from build123d import *

# Parameters (mm, degrees)
BOSS_EXTRUDE1_DEPTH = 2


with BuildPart() as part:
    # Sketch2 → Boss-Extrude1 (new body)
    with BuildSketch(Plane(origin=(0, 0, 0), x_dir=(1, 0, 0), z_dir=(0, 1, 0))):
        with BuildLine():
            Line((-3.625231148, -1.690473047), (-2.357376363, -4.409396408))
            ThreePointArc((-2.357376363, -4.409396408), (-1.93416063, -4.797202177), (-1.360681826, -4.772163552))
            Line((-1.360681826, -4.772163552), (-1.13410488, -4.666508987))
            ThreePointArc((-1.13410488, -4.666508987), (-0.96265902, -4.513901105), (-0.903326596, -4.292174896))
            Line((-0.903326596, -4.292174896), (-0.941712266, -2.992741735))
            ThreePointArc((-0.941712266, -2.992741735), (-1.04172473, -2.435992925), (-1.3, -1.932737905))
            ThreePointArc((-1.3, -1.932737905), (0, 0.6), (1.3, -1.932737905))
            ThreePointArc((1.3, -1.932737905), (1.04172473, -2.435992925), (0.941712266, -2.992741735))
            Line((0.941712266, -2.992741735), (0.903326596, -4.292174896))
            ThreePointArc((0.903326596, -4.292174896), (0.96265902, -4.513901105), (1.13410488, -4.666508987))
            Line((1.13410488, -4.666508987), (1.360681826, -4.772163552))
            ThreePointArc((1.360681826, -4.772163552), (1.93416063, -4.797202177), (2.357376363, -4.409396408))
            Line((2.357376363, -4.409396408), (3.625231148, -1.690473047))
            ThreePointArc((3.625231148, -1.690473047), (0, 4), (-3.625231148, -1.690473047))
        make_face()
    extrude(amount=BOSS_EXTRUDE1_DEPTH)


solid = part.part
Geometry: final body of the model. Coordinates: model frame, mm. A direction names the side the tool comes from. Round coordinates to 2 decimals unless told otherwise and drop trailing zeros. Loops run counter-clockwise (first coordinate to the right, second up) from the corner with the lowest first, then second, coordinate; pieces in that order, holes last.
Q1. Material intervals for L1, parallel to Z at x = 0, y = 0.9; L2, parallel to X at y = 0.9, z = 4; L3, parallel to X at y = 1.5, z = 2.75, sorted ascending.
Q2. Section B-B on y = 0.9. Return loops of the section in (x, z), plus the area to 3 significant figures.
Q3. Access query for faces 4 (the cylindrical face through (1.044, 0.986, 2.428)), 5 (the flat face through (0, 0, -1)). Directions: +Z, -Z, +X, -X, +Y, -Y. A direction counts if a zero-diameter tool reaches every point of the face in a straight line with its end or side. Return the directions, or none.
Q4. Pull-direction query (Z, two-part tool) for faces 1 (the cylindrical face through (1.93, 0.99, 4.8)), 2 (the cylindrical face through (0, 1, -0.6)), 3 (the flat face through (0, 2, -1)); classes: released by +Z, released by -Z, zero draft, split by the parting line, or undercut.
Q5. Section D-D on z = 0. Return loops of the section in (x, y).
Q6. Section A-A on z = 3.25. Return loops of the section in (x, y), plus the area to 3 significant figures.
Q7. Section C-C on x = 0. Return loops of the section in (y, z).
Evaluation:
1. L1: z = -4 to -0.6
1. L2: x = -2.55 to -0.91, 0.91 to 2.55
1. L3: x = -3.13 to -0.96, 0.96 to 3.13
2. outline: (-3.63, 1.69) arc R4 ccw (long way) to (3.63, 1.69) - (2.36, 4.41) arc R0.75 ccw to (1.36, 4.77) - (1.13, 4.67) arc R0.4 ccw to (0.9, 4.29) - (0.94, 2.99) arc R1.92 ccw to (1.3, 1.93) arc R1.6 cw (long way) to (-1.3, 1.93) arc R1.92 ccw to (-0.94, 2.99) - (-0.9, 4.29) arc R0.4 ccw to (-1.13, 4.67) - (-1.36, 4.77) arc R0.75 ccw to (-2.36, 4.41) - close
2. area: 43.7 mm2
3. face 4: +Y, -Y
3. face 5: +Z, -Z, +X, -X, -Y
4. face 1: released by +Z
4. face 2: undercut
4. face 3: zero draft
5. outline: (-4, 0) - (-1.25, 0) - (-1.25, 2) - (-4, 2) - close; (1.25, 0) - (4, 0) - (4, 2) - (1.25, 2) - close
6. outline: (-2.9, 0) - (-0.93, 0) - (-0.93, 2) - (-2.9, 2) - close; (0.93, 0) - (2.9, 0) - (2.9, 2) - (0.93, 2) - close
6. area: 7.86 mm2
7. outline: (0, -4) - (2, -4) - (2, -0.6) - (0, -0.6) - close
